Source: CAD feature listing. Evaluate the final solid. Frame: model axes, mm. A direction names the side the tool comes from. Round coordinates to 2 decimals unless told otherwise and drop trailing zeros. Loops run counter-clockwise (first coordinate to the right, second up) from the corner with the lowest first, then second, coordinate; pieces in that order, holes last. Notation, with made-up numbers: M 19.25,81 L 60.25,81 A18 ccw 60.25,99 Z; hole C -30.75,-13 d8. An arc over 180 degrees is marked long. Write each question's results on one line, items separated by ' | '. Start each with the question number.
1. Draft query along Y for faces 3 (the cylindrical face through (-112, -119.83, 3.22)), 4 (the flat face through (-98, -159.642, 3)), 5 (the flat face through (-98, -108, 6.35)). Return one class per face: released by +Y, released by -Y, zero draft, split by the parting line, or undercut.
2. Section D-D on x = -109.5. Output: boundary loops of the cut face in (y, z).
3. Set-up query: faces 1 (the flat face through (-74.992, -84, 3)), 2 (the cylindrical face through (-111.154, -146.331, 3.219)). Return all of +Z, -Z, +X, -X, +Y, -Y with unobstructed straight access to the full face (end or side cutting, diameter ignored); none if empty.
4. Section B-B on z = 3.5. Give the number of separate pieces and of enclosed holes in the cut face, and give its area (3 significant figures).
5. Section A-A on x = -94. Output: boundary loops of the cut face in (y, z), and give its area (3 significant figures).
6. Contact query for flat-ended pins moving along their axis: pin 1 Ø23 at (x, y) = (-100.39, -80.48) entering from -Z; pin 2 Ø3 at (x, z) = (-73, 2) entering from +Y. Output: stop coordinate, or through.
7. Section C-C on x = -88. Output: boundary loops of the cut face in (y, z), and give its area (3 significant figures).
8. Ray query, line 1 (Y direction, x = -100.5, z = 0.5); line 2 (Y direction, x = -76, z = 5.75); line 3 (X direction, y = -123, z = 5). Return the intervals inside material, ascending.
from build123d import *

# Parameters (mm, degrees)
BOSS_EXTRUDE1_DEPTH = 6.35
SKETCH3_R           = 14.2875
SKETCH3_R_2         = 2.032
CUT_EXTRUDE1_DEPTH  = 6.35


with BuildPart() as part:
    # Sketch2 → Boss-Extrude1 (new body)
    with BuildSketch(Plane.XY):
        Polygon((-125.79203122, -159.641560721), (-74.99203122, -159.641560721), (-68.64203122, -159.641560721), (-68.64203122, -108.841560721), (-74.99203122, -108.841560721), (-74.99203122, -58.041560721), (-125.79203122, -58.041560721), align=None)
    extrude(amount=BOSS_EXTRUDE1_DEPTH)

    # Sketch3 → Cut-Extrude1 (cut)
    with BuildSketch(Plane.XY.offset(6.35)):
        with Locations((-100.39203122, -80.483788015)):
            Circle(SKETCH3_R)
        with Locations((-87.69203122, -146.941560721)):
            Circle(SKETCH3_R_2)
        with Locations((-113.09203122, -146.941560721)):
            Circle(SKETCH3_R_2)
        with Locations((-100.39203122, -146.941560721)):
            Circle(SKETCH3_R_2)
        with Locations((-74.99203122, -146.941560721)):
            Circle(SKETCH3_R_2)
        with Locations((-113.09203122, -121.541560721)):
            Circle(SKETCH3_R_2)
        with Locations((-87.69203122, -121.541560721)):
            Circle(SKETCH3_R_2)
        with Locations((-74.99203122, -121.541560721)):
            Circle(SKETCH3_R_2)
        with Locations((-100.39203122, -121.541560721)):
            Circle(SKETCH3_R_2)
    extrude(amount=-CUT_EXTRUDE1_DEPTH, mode=Mode.SUBTRACT)


solid = part.part
Taken from the geometry:
1) face 3: undercut | face 4: released by -Y | face 5: zero draft
2) outline: M -159.64,0 L -91.49,0 L -91.49,6.35 L -159.64,6.35 Z; M -69.48,0 L -58.04,0 L -58.04,6.35 L -69.48,6.35 Z
3) face 1: +Z, -Z, +X, +Y | face 2: +Z, -Z
4) separate pieces: 1 | enclosed holes: 9 | area: 4,740 mm^2
5) outline: M -159.64,0 L -93.26,0 L -93.26,6.35 L -159.64,6.35 Z; M -67.71,0 L -58.04,0 L -58.04,6.35 L -67.71,6.35 Z | area: 483 mm^2
6) pin 1: through | pin 2: y = -108.84
7) outline: M -159.64,0 L -148.95,0 L -148.95,6.35 L -159.64,6.35 Z; M -144.93,0 L -123.55,0 L -123.55,6.35 L -144.93,6.35 Z; M -119.53,0 L -87.6,0 L -87.6,6.35 L -119.53,6.35 Z; M -73.37,0 L -58.04,0 L -58.04,6.35 L -73.37,6.35 Z | area: 504 mm^2
8) line 1: -159.64 to -148.97, -144.91 to -123.57, -119.51 to -94.77, -66.2 to -58.04 | line 2: -159.64 to -148.71, -145.18 to -123.31, -119.78 to -58.04 | line 3: -125.79 to -114.51, -111.68 to -101.81, -98.98 to -89.11, -86.28 to -76.41, -73.58 to -68.64
